Autodesk Inventor part; units mm, degrees
ref_plane "YZ Plane" through (0, 0, 0) normal (1, 0, 0) x (0, 1, 0)
ref_plane "XZ Plane" through (0, 0, 0) normal (0, 1, 0) x (-1, 0, 0)
ref_plane "XY Plane" through (0, 0, 0) normal (0, 0, 1) x (1, 0, 0)
sketch "Sketch1" plane through (0, 0, 0) normal (0, 1, 0) x (-1, 0, 0)
  line L0 (0, 0) -> (-3.175, 0)
  line L1 (-3.175, 0) -> (-3.175, 152.4)
  line L2 (-3.175, 152.4) -> (0, 152.4)
  line L3 (0, 152.4) -> (0, 0)
  dimension "d0" = 3.175
  dimension "d1" = 152.4
extrude "Extrusion1" add sketch "Sketch1" along normal blind 50.8
sketch "Sketch2" plane through (0, 0, 0) normal (0, -1, 0) x (1, 0, 0)
  line L0 (0, 0) -> (127, 0) construction
  line L1 (0, 0) -> (127, 0) construction
  line L2 (127, 0) -> (123.825, 0)
  line L3 (123.825, 0) -> (123.825, 152.4)
  line L4 (123.825, 152.4) -> (127, 152.4)
  line L5 (127, 152.4) -> (127, 0)
  dimension "d4" = 127
  dimension "d5" = 0
  dimension "d6" = 3.175
  dimension "d7" = 152.4
extrude "Extrusion2" add sketch "Sketch2" against normal blind 50.8
sketch "Sketch3" plane through (0, 0, 152.4) normal (0, 0, 1) x (1, 0, 0)
  line L0 (3.175, 0) -> (3.175, 50.8)
  line L1 (3.175, 0) -> (15.875, 0)
  line L2 (15.875, 0) -> (15.875, 3.175)
  line L3 (15.875, 3.175) -> (3.175, 3.175)
  line L4 (3.175, 3.175) -> (3.175, 0)
  point P0 (0, 0)
  point P1 (3.175, 3.175)
  dimension "d10" = 12.7
  dimension "d11" = 3.175
extrude "Extrusion3" add sketch "Sketch3" against normal blind 152.4
sketch "Sketch4" plane through (123.825, 0, 152.4) normal (0, 0, 1) x (1, 0, 0)
  line L0 (0, 0) -> (0, 50.8)
  line L1 (0, 0) -> (-12.7, 0)
  line L2 (-12.7, 0) -> (-12.7, 3.175)
  line L3 (-12.7, 3.175) -> (0, 3.175)
  line L4 (0, 3.175) -> (0, 0)
  point P0 (-123.825, 0)
  dimension "d14" = 12.7
  dimension "d15" = 3.175
extrude "Extrusion4" add sketch "Sketch4" against normal blind 152.4
sketch "Sketch5" plane through (0, 50.8, 152.4) normal (0, 0, 1) x (1, 0, 0)
  line L0 (15.875, -47.625) -> (3.175, -47.625) construction
  line L1 (3.175, -47.625) -> (3.175, -42.545) construction
  line L2 (3.175, -47.625) -> (3.175, 0) construction
  line L3 (127, 0) -> (123.825, 0)
  line L4 (3.175, -42.545) -> (123.825, -42.545)
  line L5 (123.825, -42.545) -> (123.825, 0)
  line L6 (123.825, 0) -> (3.175, 0)
  line L7 (3.175, 0) -> (3.175, -42.545)
  point P0 (0, -50.8)
  dimension "d18" = 5.08
extrude "Extrusion5" add sketch "Sketch5" against normal blind 3.175
sketch "Sketch6" plane through (127, 50.8, 0) normal (0, 0, -1) x (-1, 0, 0)
  line L0 (0, 0) -> (3.175, 0)
  line L1 (123.825, -42.545) -> (3.175, -42.545)
  line L2 (3.175, 0) -> (123.825, 0)
  line L3 (123.825, 0) -> (123.825, -42.545)
  line L4 (123.825, -42.545) -> (3.175, -42.545)
  line L5 (3.175, -42.545) -> (3.175, 0)
  point P0 (127, -50.8)
extrude "Extrusion6" add sketch "Sketch6" against normal blind 3.175
sketch "Sketch8" plane through (3.175, 3.175, 152.4) normal (1, 0, 0) x (0, 0, -1)
  line L0 (3.175, 47.625) -> (53.975, 47.625) construction
  line L1 (3.175, 47.625) -> (149.225, 47.625) construction
  line L2 (3.175, 47.625) -> (53.975, 47.625) construction
  line L3 (152.4, -3.175) -> (0, -3.175) construction
  line L4 (53.975, 47.625) -> (101.6, 47.625) construction
  line L5 (53.975, 0) -> (53.975, 5.08) construction
  line L6 (53.975, 47.625) -> (53.975, 5.08) construction
  line L7 (52.3875, 47.625) -> (55.5625, 47.625)
  line L8 (55.5625, 47.625) -> (55.5625, 5.08)
  line L9 (55.5625, 5.08) -> (52.3875, 5.08)
  line L10 (52.3875, 5.08) -> (52.3875, 47.625)
  line L11 (52.3875, 47.625) -> (55.5625, 5.08) construction
  line L12 (55.5625, 47.625) -> (52.3875, 5.08) construction
  point P0 (53.975, 26.3525)
  dimension "d26" = 50.8
  dimension "d27" = 0
  dimension "d28" = 47.625
  dimension "d30" = 5.08
  dimension "d32" = 3.175
extrude "Extrusion7" add sketch "Sketch8" along normal up to next
sketch "Sketch9" plane through (3.175, 3.175, 152.4) normal (1, 0, 0) x (0, 0, -1)
  line L0 (149.225, 5.08) -> (149.225, 47.625) construction
  line L1 (149.225, 47.625) -> (98.425, 47.625) construction
  line L2 (55.5625, 47.625) -> (149.225, 47.625) construction
  line L3 (98.425, 47.625) -> (146.05, 47.625) construction
  line L4 (98.425, 0) -> (98.425, 5.08) construction
  line L5 (98.425, 47.625) -> (98.425, 5.08) construction
  line L6 (96.8375, 47.625) -> (100.0125, 47.625)
  line L7 (100.0125, 47.625) -> (100.0125, 5.08)
  line L8 (100.0125, 5.08) -> (96.8375, 5.08)
  line L9 (96.8375, 5.08) -> (96.8375, 47.625)
  line L10 (96.8375, 47.625) -> (100.0125, 5.08) construction
  line L11 (100.0125, 47.625) -> (96.8375, 5.08) construction
  point P0 (152.4, -3.175)
  point P1 (98.425, 26.3525)
  dimension "d35" = 50.8
  dimension "d36" = 47.625
  dimension "d38" = 5.08
  dimension "d40" = 3.175
  dimension "d41" = 42.545
extrude "Extrusion8" add sketch "Sketch9" along normal up to next
sketch "Sketch10" plane through (0, 50.8, 0) normal (0, 1, 0) x (1, 0, 0)
  line L0 (3.175, -55.5625) -> (123.825, -55.5625) construction
  line L1 (123.825, -55.5625) -> (127, -55.5625) construction
  line L2 (127, 0) -> (127, -152.4) construction
  line L3 (3.175, -100.0125) -> (123.825, -100.0125) construction
  line L4 (3.175, -100.0125) -> (0, -100.0125) construction
  line L5 (127, 0) -> (0, 0)
  line L6 (0, 0) -> (127, 0)
  line L7 (127, 0) -> (127, -55.5625)
  line L8 (127, -55.5625) -> (0, -55.5625)
  line L9 (0, -55.5625) -> (0, 0)
  line L10 (3.175, -3.175) -> (123.825, -3.175)
  line L11 (123.825, -3.175) -> (123.825, -52.3875)
  line L12 (123.825, -52.3875) -> (3.175, -52.3875)
  line L13 (3.175, -52.3875) -> (3.175, -3.175)
  line L14 (0, -100.0125) -> (127, -100.0125)
  line L15 (127, -100.0125) -> (127, -52.3875)
  line L16 (127, -52.3875) -> (0, -52.3875)
  line L17 (0, -52.3875) -> (0, -100.0125)
  line L18 (3.175, -96.8375) -> (123.825, -96.8375)
  line L19 (123.825, -96.8375) -> (123.825, -55.5625)
  line L20 (123.825, -55.5625) -> (3.175, -55.5625)
  line L21 (3.175, -55.5625) -> (3.175, -96.8375)
  line L22 (0, 0) -> (0, -152.4)
  line L23 (0, -152.4) -> (127, -152.4)
  line L24 (127, -152.4) -> (127, -96.8375)
  line L25 (127, -96.8375) -> (0, -96.8375)
  line L26 (0, -96.8375) -> (0, -152.4)
  line L27 (123.825, -149.225) -> (3.175, -149.225)
  line L28 (3.175, -149.225) -> (3.175, -100.0125)
  line L29 (3.175, -100.0125) -> (123.825, -100.0125)
  line L30 (123.825, -100.0125) -> (123.825, -149.225)
  point P0 (3.175, -55.5625)
  dimension "d44" = 3.175
  dimension "d45" = 3.175
  dimension "d46" = 3.175
extrude "Extrusion9" add sketch "Sketch10" along normal blind 50.8 contours L7 L16 L11 L10 L13 L9 L5 | L7 L8 L9 L16 L12 | L15 L25 L19 L8 | L8 L21 L25 L17 | L15 L14 L17 L25 L18 | L24 L23 L22 L14 L28 L27 L30
properties part number "BeadCompartments_1"
Geometry check sheet. Reference: the model listing, model coordinates, mm. A direction names the side the tool comes from. Give positions to 0.01 mm unless a question says otherwise; leave off trailing zeros. Loops run counter-clockwise (first coordinate to the right, second up) from the corner with the lowest first, then second, coordinate; pieces in that order, holes last. Notation, with made-up numbers: (24.25, -23) - (62.25, -23) arc R14 cw to (62.25, -5) - close; hole circle Ø9 at (-17.75, 34.5). An arc over 180 degrees is marked (long way). Use CSV: the item, a comma, the result in double quotes. Start each with the question number.
Q1. Section check C-C, the plane x = 105.5. Record the cut outline in (y, z) (1 decimal), and give its area (3 significant figures).
Q2. Scan lines: probe 1 along Z at (x, y) = (15, 17.5) (1 decimal); probe 2 along X at (y, z) = (78, 36) (3 decimals); probe 3 along Y at (x, z) = (115, 10) (3 decimals). Record each from-to range of solid material in increasing order. Write a range as from..to.
Q3. Release check for a two-part mould opening along X. For faces 1 (the face through (8, 0, 77)), 2 (the face through (127, 50, 77)), 3 (the face through (10, 3.175, 77)) record: +X half, -X half, draft (parallel to the pull), parting line (faces both ways), or undercut.
Q4. Access from +Z, -Z, +X, -X, +Y, -Y to the whole of each face (thin tool, end or side, straight path). Record for faces 4 (the face through (119, 0, 77)), 5 (the face through (63, 54, 100.012)).
Q5. Go/stop test with flat-tipped pins: pin 1 Ø6.5 at (x, z) = (7.5, 45.5) entering from +Y (3 decimals); pin 2 Ø1.6 at (x, z) = (91, 2.5) entering from -Y (3 decimals). Record where each tip stops, or that it passes through.
Q6. Section check B-B, the plane z = 24.5. Record the cut outline in (x, y) (3 decimals), and give its area (3 significant figures).
Q7. Section check A-A, the plane x = 8.5. Record the cut outline in (y, z) (1 decimal).
Q8. Section check D-D, the plane y = 57. Record the cut outline in (x, z) (1 decimal), and give its area (3 significant figures).
Findings below:
1,outline,"(8.3, 0) - (101.6, 0) - (101.6, 3.2) - (8.3, 3.2) - close; (8.3, 52.4) - (101.6, 52.4) - (101.6, 55.6) - (8.3, 55.6) - close; (8.3, 96.8) - (101.6, 96.8) - (101.6, 100) - (8.3, 100) - close; (8.3, 149.2) - (101.6, 149.2) - (101.6, 152.4) - (8.3, 152.4) - close"
1,area,"1,190 mm^2"
2,probe 1,"z = 0..3.2, 52.4..55.6, 96.8..100, 149.2..152.4"
2,probe 2,"x = 0..3.175, 123.825..127"
2,probe 3,"y = 0..3.175"
3,face 1,"draft"
3,face 2,"+X half"
3,face 3,"undercut"
4,face 4,"+Z, -Z, +X, -X, -Y"
4,face 5,"+Y"
5,pin 1,"stops at y = 3.175"
5,pin 2,"stops at y = 8.255"
6,outline,"(0, 0) - (15.875, 0) - (15.875, 3.175) - (3.175, 3.175) - (3.175, 101.6) - (0, 101.6) - close; (111.125, 0) - (127, 0) - (127, 101.6) - (123.825, 101.6) - (123.825, 3.175) - (111.125, 3.175) - close"
6,area,"726 mm^2"
7,outline,"(0, 0) - (3.2, 0) - (3.2, 152.4) - (0, 152.4) - close; (8.3, 0) - (101.6, 0) - (101.6, 3.2) - (8.3, 3.2) - close; (8.3, 52.4) - (101.6, 52.4) - (101.6, 55.6) - (8.3, 55.6) - close; (8.3, 96.8) - (101.6, 96.8) - (101.6, 100) - (8.3, 100) - close; (8.3, 149.2) - (101.6, 149.2) - (101.6, 152.4) - (8.3, 152.4) - close"
8,outline,"(0, 0) - (127, 0) - (127, 152.4) - (0, 152.4) - close; hole (3.2, 3.2) - (123.8, 3.2) - (123.8, 52.4) - (3.2, 52.4) - close; hole (3.2, 55.6) - (123.8, 55.6) - (123.8, 96.8) - (3.2, 96.8) - close; hole (3.2, 100) - (123.8, 100) - (123.8, 149.2) - (3.2, 149.2) - close"
8,area,"2,500 mm^2"
